CAD build for the part. Positions are in the model's coordinates, mm. Give positions to 0.01 mm unless a question says otherwise; leave off trailing zeros. Write each loop counter-clockwise with the first axis right and the second up, starting at its lowest first coordinate (ties: lowest second). Pieces come first, ordered by that corner, then holes. Notation, with made-up numbers: (67.25, -39.5) - (82.25, -39.5) arc R15 cw to (82.25, -27.5) - close; hole circle Ø5 at (63.25, 56). An arc over 180 degrees is marked (long way). Answer as a JSON object with one key per item and string values.
from build123d import *

# Parameters (mm, degrees)
SKETCH2_R           = 2
BOSS_EXTRUDE1_DEPTH = 5
CHAMFER2_SIZE       = 1


with BuildPart() as part:
    # Sketch2 → Boss-Extrude1 (new body)
    with BuildSketch(Plane.XY):
        Polygon((-33.204562103, 16.96373801), (-38.977999735, 16.936329175), (-41.840981804, 11.922681101), (-38.93052624, 6.936441863), (-33.157088608, 6.963850698), (-30.29410654, 11.977498771), align=None)
        with Locations((-36.067544172, 11.950089936)):
            Circle(SKETCH2_R, mode=Mode.SUBTRACT)
    extrude(amount=BOSS_EXTRUDE1_DEPTH)

    # Chamfer2
    chamfer2_edges = [part.edges().sort_by_distance(p)[0] for p in [
        (-40.409490769, 14.429505138, 5),
        (-40.385754022, 9.429561482, 5),
        (-38.067544172, 11.950089936, 0),
        (-38.067544172, 11.950089936, 5),
        (-36.043807424, 6.95014628, 5),
        (-31.725597574, 9.470674734, 5),
        (-31.749334322, 14.470618391, 5),
        (-31.725597574, 9.470674734, 0),
        (-36.043807424, 6.95014628, 0),
        (-40.385754022, 9.429561482, 0),
        (-40.409490769, 14.429505138, 0),
        (-36.091280919, 16.950033593, 0),
        (-31.749334322, 14.470618391, 0),
        (-36.091280919, 16.950033593, 5),
    ]]
    chamfer(chamfer2_edges, length=CHAMFER2_SIZE)


solid = part.part
Item 1: Cut at A-A (z = 4.65). Give the cut face in (x, y), and give its area (3 significant figures).
Entries:
{"outline": "(-41.09, 11.93) - (-38.56, 7.59) - (-33.54, 7.61) - (-31.04, 11.97) - (-33.58, 16.31) - (-38.6, 16.29) - close; hole circle Ø5.3 at (-36.07, 11.95)", "area": "43.5 mm2"}
Item 2: Flat gauge pins, fed straight in: P1, Ø3, axis at x = -31.5, z = 1.5, coming from the +Y side; P2, Ø1, axis at x = -33, z = 2, coming from the +Y side; P3, Ø2, axis at y = 14.5, z = 4, coming from the -X side; P4, Ø1.5, axis at x = -36, z = 3, coming from the -Y side. Where does each tip first touch, or does it go through?
Entries:
{"P1": "y = 16.61", "P2": "y = 16.96", "P3": "x = -40.94", "P4": "y = 6.95"}
Item 3: Cut at D-D (z = 1.3). Give the cut face in (x, y), and give its area (3 significant figures).
Entries:
{"outline": "(-41.84, 11.92) - (-38.93, 6.94) - (-33.16, 6.96) - (-30.29, 11.98) - (-33.2, 16.96) - (-38.98, 16.94) - close; hole circle Ø4 at (-36.07, 11.95)", "area": "74.0 mm2"}
Item 4: Mould opens along Y. For faces 1 (the flat face through (-33, 11, 5)), 2 (the flat face through (-39.95, 14.21, 4.51)), 3 (the flat face through (-40.406, 9.464, 2.479)), 4 (the cylindrical face through (-36.501, 9.998, 2.479)) say: +Y half, -Y half, draft (parallel to the pull), parting line (faces both ways), or undercut.
Entries:
{"face 1": "draft", "face 2": "+Y half", "face 3": "-Y half", "face 4": "undercut"}
Item 5: Probe line 1 (X direction, y = 13.75, z = 1.2); line 2 (Y direction, x = -36.5, z = 3.15); line 3 (X direction, y = 12.25, z = 0.8). List the from-to ranges inside material, lowest first. Write a range as from..to.
Entries:
{"line 1": "-40.8..-36.94, -35.2..-31.33", "line 2": "6.95..10, 13.9..16.95", "line 3": "-41.42..-38.25, -33.89..-30.68"}
Item 6: Cut at B-B (y = 15.75). Give the cut face in (x, z).
Entries:
{"outline": "(-39.66, 1) - (-38.5, 0) - (-33.65, 0) - (-32.5, 1) - (-32.5, 4) - (-33.65, 5) - (-38.5, 5) - (-39.66, 4) - close"}
Item 7: Cut at C-C (x = -39.25). Give the cut face in (y, z), and give its area (3 significant figures).
Entries:
{"outline": "(7.48, 1) - (9.47, 0) - (14.44, 0) - (16.46, 1) - (16.46, 4) - (14.44, 5) - (9.47, 5) - (7.48, 4) - close", "area": "40.9 mm2"}
